Read the model definition and answer for the solid it produces. Units are mm, in the model's axes. A direction names the side the tool comes from. Coordinates: 2 decimals unless noted, no trailing zeros. Loops run counter-clockwise (first coordinate to the right, second up) from the corner with the lowest first, then second, coordinate; pieces in that order, holes last. Notation, with made-up numbers: (54, -13.5) -> (59, -13.5) arc R20 ccw to (59, 22.5) -> close; hole circle Ø2 at (68, 16). An arc over 180 degrees is marked (long way). Answer as a JSON object with one key per item and string values. Group by question number.
Q1. The part is cut by section C-C on z = 62. Write down the section's boundary in (x, y), and give its area (3 significant figures).
Q2. For faces 1 (the cylindrical face through (95.38, 30.04, 415.04)), 2 (the cylindrical face through (39.054, 297.447, 1.54)), determine the directions among +Z, -Z, +X, -X, +Y, -Y from which every point of the face is accessible in a straight line to the end or side of a thin tool.
Q3. Each of these flat-tipped pins is pushed along its axis until it touches: P1, Ø12, axis at y = 133.5, z = -25.5, coming from the +X side; P2, Ø12, axis at x = -26.5, z = 58.5, coming from the +Y side; P3, Ø2, axis at x = 186, z = 85.5, coming from the -Y side. Where does it stop, or does it pass through?
Q4. Straight lines are drawn through the part: line 1 along X through (y, z) = (-43, 376); line 2 along X through (y, z) = (-217, 13); line 3 along Y through (x, z) = (156.5, 101.5). For each, find the intervals that lie inside material, in ascending order. Write a range as [from, to].
from build123d import *

# Parameters (mm, degrees)
BOSS_EXTRUDE1_DEPTH      = 250
BOSS_EXTRUDE1_DEPTH_BACK = 250
SKETCH1_R                = 100
SKETCH2_R                = 300
BOSS_EXTRUDE2_DEPTH      = 220
CHAMFER1_SIZE2           = 115.470053838
CHAMFER1_SIZE            = 200


with BuildPart() as part:
    # Sketch1 → Boss-Extrude1 (new, two sides: drawn at the far end of the back side and taken through both)
    with BuildSketch(Plane.XY.offset(-BOSS_EXTRUDE1_DEPTH_BACK)):
        Circle(SKETCH1_R)
    extrude(amount=BOSS_EXTRUDE1_DEPTH + BOSS_EXTRUDE1_DEPTH_BACK)

    # Sketch2 → Boss-Extrude2 (add)
    with BuildSketch(Plane(origin=(0, 0, -250), x_dir=(-1, 0, 0), z_dir=(0, 0, -1))):
        Circle(SKETCH2_R)
    extrude(amount=BOSS_EXTRUDE2_DEPTH)

    # Chamfer1
    chamfer1_edges = [part.edges().sort_by_distance(p)[0] for p in [
        (-100, 0, -250),
    ]]
    chamfer1_side = [part.faces().sort_by_distance(p)[0] for p in [
        (-102.309401077, 0, -250),
    ]]
    chamfer(chamfer1_edges, length=CHAMFER1_SIZE - 0.0001, length2=CHAMFER1_SIZE2 - 0.0001, reference=chamfer1_side[0])  # a hair under: the kernel refuses the full size


with BuildPart() as part_1:
    # Body-Move/Copy1: moved
    add(part.part.moved(Location((0, 0, 360))))


solid = part_1.part
Final values:
{
 "1": {"outline": "circle Ø600 at (0, 0)", "area": "283,000 mm2"},
 "2": {"face 1": "+Z", "face 2": "+Z, -Z"},
 "3": {"P1": "stops at x = 271.56", "P2": "stops at y = 299.3", "P3": "stops at y = -236.17"},
 "4": {"line 1": "x = [-90.28, 90.28]", "line 2": "x = [-207.15, 207.15]", "line 3": "y = [-255.94, 255.94]"}
}
